```python
from build123d import *

# Parameters (mm, degrees)
BOSS_EXTRUDE1_DEPTH = 304.8
FILLET2_R           = 2.54
FILLET7_R           = 0.762


with BuildPart() as part:
    # Sketch1 → Boss-Extrude1 (new body)
    with BuildSketch(Plane.XY):
        with BuildLine():
            Line((-59.991213716, 144.035687339), (-8.193810242, 180.296949153))
            ThreePointArc((-8.193810242, 180.296949153), (0, 182.88), (8.193810242, 180.296949153))
            Line((8.193810242, 180.296949153), (59.991213716, 144.035687339))
            add(Edge.make_bspline(
                [(59.991213716, 144.035687339), (62.78248672, 142.0840471), (62.441206007, 139.021062406)],
                knots=[0, 0, 0, 1, 1, 1], degree=2))
            ThreePointArc((62.441206007, 139.021062406), (51.81191727, 143.32231239), (40.889317917, 146.812205488))
            Line((40.889317917, 146.812205488), (42.636417316, 149.30784982))
            Line((42.636417316, 149.30784982), (44.875008407, 148.34072044))
            Line((44.875008407, 148.34072044), (45.552343011, 149.308259131))
            add(Edge.make_bspline(
                [(45.552343011, 149.308259131), (43.180649259, 153.803743217), (38.144971739, 154.493859392)],
                knots=[0, 0, 0, 1, 1, 1], degree=2))
            Line((38.144971739, 154.493859392), (37.467637136, 153.526320702))
            Line((37.467637136, 153.526320702), (39.142437036, 151.753843735))
            Line((39.142437036, 151.753843735), (36.49122578, 147.966720721))
            ThreePointArc((36.49122578, 147.966720721), (31.806362047, 149.044004688), (27.089852549, 149.972997199))
            Line((27.089852549, 149.972997199), (33.300728714, 158.844923948))
            Line((33.300728714, 158.844923948), (6.372963522, 177.695960452))
            ThreePointArc((6.372963522, 177.695960452), (0, 179.705), (-6.372963522, 177.695960452))
            Line((-6.372963522, 177.695960452), (-33.300728714, 158.844923948))
            Line((-33.300728714, 158.844923948), (-27.089852549, 149.972997199))
            ThreePointArc((-27.089852549, 149.972997199), (-31.806362047, 149.044004688), (-36.49122578, 147.966720721))
            Line((-36.49122578, 147.966720721), (-39.142437036, 151.753843735))
            Line((-39.142437036, 151.753843735), (-37.467637136, 153.526320702))
            Line((-37.467637136, 153.526320702), (-38.144971739, 154.493859392))
            add(Edge.make_bspline(
                [(-45.552343011, 149.308259131), (-43.180649259, 153.803743217), (-38.144971739, 154.493859392)],
                knots=[0, 0, 0, 1, 1, 1], degree=2))
            Line((-45.552343011, 149.308259131), (-44.875008407, 148.34072044))
            Line((-44.875008407, 148.34072044), (-42.636417316, 149.30784982))
            Line((-42.636417316, 149.30784982), (-40.889317917, 146.812205488))
            ThreePointArc((-40.889317917, 146.812205488), (-51.81191727, 143.32231239), (-62.441206007, 139.021062406))
            add(Edge.make_bspline(
                [(-59.991213716, 144.035687339), (-62.78248672, 142.0840471), (-62.441206007, 139.021062406)],
                knots=[0, 0, 0, 1, 1, 1], degree=2))
        make_face()
    extrude(amount=BOSS_EXTRUDE1_DEPTH)

    # Fillet2
    fillet2_edges = [part.edges().sort_by_distance(p)[0] for p in [
        (33.300728714, 158.844923948, 152.4),
        (-33.300728714, 158.844923948, 152.4),
    ]]
    fillet(fillet2_edges, radius=FILLET2_R)

    # Fillet7
    fillet7_edges = [part.edges().sort_by_distance(p)[0] for p in [
        (40.889317917, 146.812205488, 152.4),
        (36.49122578, 147.966720721, 152.4),
        (27.089852549, 149.972997199, 152.4),
        (-27.089852549, 149.972997199, 152.4),
        (-36.49122578, 147.966720721, 152.4),
        (-40.889317917, 146.812205488, 152.4),
    ]]
    fillet(fillet7_edges, radius=FILLET7_R)


solid = part.part
```
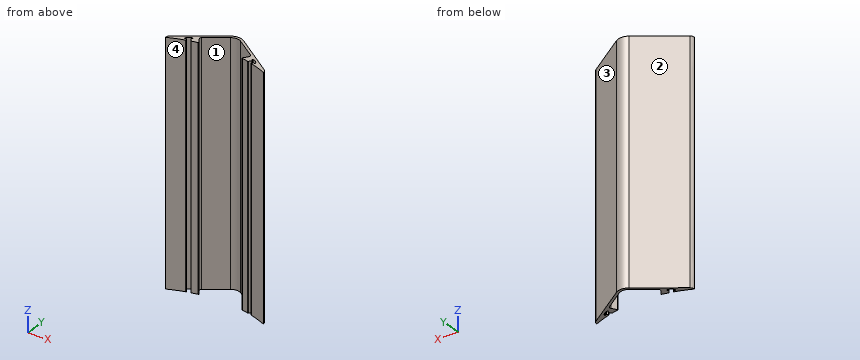
Geometry check sheet. Reference: the model listing, model coordinates, mm. Face numbers are marked on the shaded views. Coordinates: 2 decimals unless noted, no trailing zeros. Order: outer loops, then holes, each group sorted by start corner. A loop starts at its lowest first (then second) coordinate and runs counter-clockwise, first axis right, second up. Notation, with made-up numbers: M 50.5,-16 L 69.5,-16 A18 cw 69.5,-2 Z; hole C 6.5,1.25 d5. An arc over 180 degrees is marked long. Answer as a JSON object with one key per item and string values.
Q1. Cross-section at C-C on x = 14.5. Record the cut outline in (y, z), and give its area (3 significant figures).
Results are:
{"outline": "M 172.01,0 L 175.88,0 L 175.88,304.8 L 172.01,304.8 Z", "area": "1,180 mm²"}
Q2. Cross-section at A-A on y = 163. Record the cut outline in (x, z), and give its area (3 significant figures).
Results are:
{"outline": "M -32.9,0 L -27.37,0 L -27.37,304.8 L -32.9,304.8 Z; M 27.37,0 L 32.9,0 L 32.9,304.8 L 27.37,304.8 Z", "area": "3,370 mm²"}
Q3. Depth check by flat-ended pin: pin 1 Ø12 at (y, z) = (148.5, 105.5) entering from +X; pin 2 Ø5 at (y, z) = (157, 42) entering from -X; pin 3 Ø10 at (y, z) = (166.5, 84.5) entering from -X. Enter the tip coordinate at first touch or a pass-through.
Results are:
{"pin 1": "stops at x = 61.59", "pin 2": "stops at x = -45.04", "pin 3": "stops at x = -35.04"}
Q4. Scan lines: line 1 (Y direction, x = -31.5, z = 275.5); line 2 (X direction, y = 153, z = 122); line 3 (Y direction, x = -38, z = 94). Record each from-to range of solid material in increasing order.
Results are:
{"line 1": "y = 149.11 to 156.27, 160.07 to 163.98", "line 2": "x = -47.19 to -42.3, -37.96 to -29.21, 29.21 to 37.96, 42.3 to 47.19", "line 3": "y = 150.12 to 152.96, 154.29 to 159.43"}
Q5. Release check for a two-part mould opening along X. For the marked faces 1, 2, 3 and 4 record: released by +X, released by -X, zero draft, split by the parting line, or undercut.
Results are:
{"face 1": "undercut", "face 2": "released by -X", "face 3": "released by +X", "face 4": "undercut"}
Q6. Cross-section at B-B on x = -54. Record the cut outline in (y, z).
Results are:
{"outline": "M 142.51,0 L 148.23,0 L 148.23,304.8 L 142.51,304.8 Z"}
